The model under review builds one solid part; all positions refer to its coordinate system, in mm. A direction names the side the tool comes from. Give positions to 0.01 mm unless a question says otherwise; leave off trailing zeros. Loops run counter-clockwise (first coordinate to the right, second up) from the corner with the lowest first, then second, coordinate; pieces in that order, holes last. Notation, with made-up numbers: (50.5, -25) - (75.5, -25) arc R13 cw to (75.5, -4) - close; hole circle Ø2 at (34.5, 8.5). An arc over 180 degrees is marked (long way). Return JSON: item names as keys, results as strings. Group by question number.
from build123d import *

# Parameters (mm, degrees)
SKETCH2_W           = 120
SKETCH2_H           = 115
BOSS_EXTRUDE1_DEPTH = 152
SKETCH3_W           = 120
SKETCH3_H           = 13.389184999
CUT_EXTRUDE1_DEPTH  = 192.155706765
SKETCH5_R           = 3.25
CUT_EXTRUDE2_DEPTH  = 30
SKETCH6_W           = 4.5
SKETCH6_H           = 90
SKETCH6_W_2         = 106.706999447
SKETCH6_H_2         = 3.032111459
CUT_EXTRUDE4_DEPTH  = 130
SKETCH7_R           = 3.25
CUT_EXTRUDE5_DEPTH  = 15
SKETCH8_W           = 8.291807731
SKETCH8_H           = 28.961241497
SKETCH8_H_2         = 55.038375958
SKETCH8_W_2         = 108.394356143
SKETCH8_H_3         = 6.008556327
SKETCH8_W_3         = 7.690952099
SKETCH8_H_4         = 30.523466142
SKETCH8_W_4         = 6.849754213
SKETCH8_H_5         = 57.922482994
CUT_EXTRUDE6_DEPTH  = 150
CUT_EXTRUDE7_DEPTH  = 192.155706765


with BuildPart() as part:
    # Sketch2 → Boss-Extrude1 (new body)
    with BuildSketch(Plane.XY):
        with BuildLine():
            Line((-48.334664537, 64.049520767), (81.665335463, 64.049520767))
            ThreePointArc((81.665335463, 64.049520767), (88.736403275, 61.120588579), (91.665335463, 54.049520767))
            Line((91.665335463, 54.049520767), (91.665335463, -70.950479233))
            Line((91.665335463, -70.950479233), (-58.334664537, -70.950479233))
            Line((-58.334664537, -70.950479233), (-58.334664537, 54.049520767))
            ThreePointArc((-58.334664537, 54.049520767), (-55.405732349, 61.120588579), (-48.334664537, 64.049520767))
        make_face()
        with Locations((16.665335463, -3.450479233)):
            Rectangle(SKETCH2_W, SKETCH2_H, mode=Mode.SUBTRACT)
    extrude(amount=BOSS_EXTRUDE1_DEPTH)

    # Sketch3 → Cut-Extrude1 (cut, through all)
    with BuildSketch(Plane.XY.offset(152)):
        with Locations((16.665335463, -67.645071732)):
            Rectangle(SKETCH3_W, SKETCH3_H)
    extrude(amount=-CUT_EXTRUDE1_DEPTH, mode=Mode.SUBTRACT)

    # Sketch5 → Cut-Extrude2 (cut)
    with BuildSketch(Plane(origin=(0, 0, 0), x_dir=(-1, 0, 0), z_dir=(0, 0, -1))):
        with Locations((-82.665335463, 56.549520767)):
            Circle(SKETCH5_R)
        with Locations(Location((49.334664537, 56.549520767, 0), (0, 0, 180))):
            Circle(SKETCH5_R)
    extrude(amount=-CUT_EXTRUDE2_DEPTH, mode=Mode.SUBTRACT)

    # Sketch6 → Cut-Extrude4 (cut)
    with BuildSketch(Plane(origin=(0, 0, 0), x_dir=(-1, 0, 0), z_dir=(0, 0, -1))):
        with Locations((50.834664537, -0.950479233)):
            Rectangle(SKETCH6_W, SKETCH6_H)
        with Locations((-84.165335463, -0.950479233)):
            Rectangle(SKETCH6_W, SKETCH6_H)
        with Locations((-16.665335464, 59.14514242)):
            Rectangle(SKETCH6_W_2, SKETCH6_H_2)
    extrude(amount=-CUT_EXTRUDE4_DEPTH, mode=Mode.SUBTRACT)

    # Sketch7 → Cut-Extrude5 (cut)
    with BuildSketch(Plane.XY.offset(152)):
        with Locations((-50.834664537, 55.049520767)):
            Circle(SKETCH7_R)
        with Locations((-50.834664537, 4.049520767)):
            Circle(SKETCH7_R)
        with Locations(Location((84.165335463, 4.049520767, 0), (0, 0, 180))):
            Circle(SKETCH7_R)
        with Locations(Location((84.165335463, 55.049520767, 0), (0, 0, 180))):
            Circle(SKETCH7_R)
    extrude(amount=-CUT_EXTRUDE5_DEPTH, mode=Mode.SUBTRACT)

    # Sketch8 → Cut-Extrude6 (cut)
    with BuildSketch(Plane.XY.offset(152)):
        with Locations((-50.991008781, 27.795371112)):
            Rectangle(SKETCH8_W, SKETCH8_H)
        with Locations((-50.991008781, -32.350277723)):
            Rectangle(SKETCH8_W, SKETCH8_H_2)
        with Locations((16.485078773, 59.340291831)):
            Rectangle(SKETCH8_W_2, SKETCH8_H_3)
        with Locations((84.261594145, 30.258879207)):
            Rectangle(SKETCH8_W_3, SKETCH8_H_4)
        with Locations((84.682193087, -36.556267152)):
            Rectangle(SKETCH8_W_4, SKETCH8_H_5)
    extrude(amount=-CUT_EXTRUDE6_DEPTH, mode=Mode.SUBTRACT)

    # Sketch9 → Cut-Extrude7 (cut, through all)
    with BuildSketch(Plane.XY.offset(152)):
        with BuildLine():
            Line((-55.78242584, -70.950479233), (-43.00561738, -70.950479233))
            Line((-43.00561738, -70.950479233), (-43.00561738, -60.861864812))
            Line((-43.00561738, -60.861864812), (-43.334664537, -60.861864812))
            ThreePointArc((-43.334664537, -60.861864812), (-52.78845028, -61.92097783), (-55.78242584, -70.950479233))
        make_face()
    extrude(amount=-CUT_EXTRUDE7_DEPTH, mode=Mode.SUBTRACT)


solid = part.part
Item 1: Take a section at A-A (y = 27). State the section outline as (x, z) points, then the cut area to 3 significant figures.
Item 2: Take a section at D-D (y = -23). State the section outline as (x, z) points, then the cut area to 3 significant figures.
Item 3: For L1, parallel to X at y = -32, z = 48; L2, parallel to X at y = 8, z = 81; L3, parallel to Y at x = -17, z = 82, list the stretches that pass through material, from the lowest coordinate up. Write a range as from..to.
Item 4: For P1, Ø3.5, axis at x = 85, z = 56.5, coming from the +Y side; P2, Ø12, axis at x = -16, z = 101.5, coming from the -Y side; P3, Ø3, axis at x = 22, y = 59.5, coming from the +Z side, all flat-tipped, find the tip position at first contact; note any pin that passes through.
Item 5: Take a section at C-C (y = -50.5). State the section outline as (x, z) points, then the cut area to 3 significant figures.
Item 6: Take a section at B-B (x = -9.5). State the section outline as (y, z) points.
Item 7: Mouldability with a two-part tool opening along X and no side actions: class faces 5 (the face through (88.658, 61.198, 74.936)), 6 (the face through (-51, 55, 137)), 7 (the face through (16, 64.05, 75)) as +X half, -X half, draft (parallel to the pull), parting line (faces both ways), or undercut.
Item 8: Tool access review of faces 1 (the face through (-52.678, -61.833, 77.064)), 2 (the face through (76.665, -9, 75)), 3 (the face through (84, 45.521, 78)), 4 (the face through (84, 4, 130)): name each direction out of +Z, -Z, +X, -X, +Y, -Y from which nothing blocks a thin tool from reaching the whole face with its end or side.
Check sheet entries:
{
 "1": {"outline": "(-58.33, 0) - (-53.08, 0) - (-53.08, 2) - (-55.14, 2) - (-55.14, 152) - (-58.33, 152) - close; (-48.58, 0) - (-43.33, 0) - (-43.33, 152) - (-46.85, 152) - (-46.85, 2) - (-48.58, 2) - close; (76.67, 0) - (81.92, 0) - (81.92, 2) - (80.42, 2) - (80.42, 152) - (76.67, 152) - close; (86.42, 0) - (91.67, 0) - (91.67, 152) - (88.11, 152) - (88.11, 2) - (86.42, 2) - close", "area": "2,140 mm^2"},
 "2": {"outline": "(-58.33, 0) - (-53.08, 0) - (-53.08, 2) - (-55.14, 2) - (-55.14, 152) - (-58.33, 152) - close; (-48.58, 0) - (-43.33, 0) - (-43.33, 152) - (-46.85, 152) - (-46.85, 2) - (-48.58, 2) - close; (76.67, 0) - (81.92, 0) - (81.92, 2) - (81.26, 2) - (81.26, 152) - (76.67, 152) - close; (86.42, 0) - (91.67, 0) - (91.67, 152) - (88.11, 152) - (88.11, 2) - (86.42, 2) - close", "area": "2,270 mm^2"},
 "3": {"L1": "x = -58.33..-55.14, -46.85..-43.33, 76.67..81.26, 88.11..91.67", "L2": "x = -58.33..-53.08, -48.58..-43.33, 76.67..81.92, 86.42..91.67", "L3": "y = 54.05..56.34, 62.34..64.05"},
 "4": {"P1": "stops at y = 63.92", "P2": "stops at y = 54.05", "P3": "stops at z = 2"},
 "5": {"outline": "(-58.33, 0) - (-43.33, 0) - (-43.33, 152) - (-46.85, 152) - (-46.85, 2) - (-55.14, 2) - (-55.14, 152) - (-58.33, 152) - close; (76.67, 0) - (91.67, 0) - (91.67, 152) - (88.11, 152) - (88.11, 2) - (81.26, 2) - (81.26, 152) - (76.67, 152) - close", "area": "2,290 mm^2"},
 "6": {"outline": "(54.05, 0) - (57.63, 0) - (57.63, 2) - (56.34, 2) - (56.34, 152) - (54.05, 152) - close; (60.66, 0) - (64.05, 0) - (64.05, 152) - (62.34, 152) - (62.34, 2) - (60.66, 2) - close"},
 "7": {"face 5": "+X half", "face 6": "undercut", "face 7": "draft"},
 "8": {"face 1": "+Z, -Z", "face 2": "+Z, -Z, -Y", "face 3": "+Z", "face 4": "-Z"}
}
